Can you work these out from the model? Positions are in its coordinate system, mm. A direction names the side the tool comes from. Round coordinates to 2 decimals unless told otherwise and drop trailing zeros. Loops run counter-clockwise (first coordinate to the right, second up) from the corner with the lowest first, then second, coordinate; pieces in that order, holes last. Notation, with made-up numbers: (47.25, 21.25) -> (51.25, 21.25) arc R31 cw to (51.25, 50.25) -> close; hole circle Ø2 at (30.5, 84.5). An arc over 180 degrees is marked (long way). Answer as a JSON object with one key per item and string values.
```python
from build123d import *

# Parameters (mm, degrees)
F0_R     = 11.5502364961
F1_DEPTH = 76.2
F2_DEPTH = 25.4
F3_DEPTH = 25.4
F0_W     = 68.4429863468
F0_H     = 5.7512475178
F4_DEPTH = 76.2
F6_DEPTH = 25.4


with BuildPart() as f1:
    # F0 (on Top) → F1 (new body)
    with BuildSketch(Plane.XY):
        Polygon((-8.7633775547, 30.0670936704), (-48.5640950501, 30.0670936704), (-48.5640950501, -34.4098359346), (-8.7633775547, -34.4098359346), (-8.7633775547, -5.7512475178), (-8.7633775547, 0), align=None)
        with Locations((-30.1417633891, 0)):
            Circle(F0_R, mode=Mode.SUBTRACT)
    extrude(amount=F1_DEPTH)

    # F0 (on Top) → F2 (join)
    with BuildSketch(Plane.XY):
        Polygon((-8.7633775547, -5.7512475178), (-8.7633775547, -34.4098359346), (41.3302518427, -34.4098359346), (59.6796087921, -23.2587810606), (59.6796087921, -5.7512475178), align=None)
    extrude(amount=F2_DEPTH)

    # F0 (on Top) → F3 (join)
    with BuildSketch(Plane.XY):
        Polygon((41.3302518427, 30.0670936704), (-8.7633775547, 30.0670936704), (-8.7633775547, 0), (59.6796087921, 0), (59.6796087921, 18.9160387963), align=None)
    extrude(amount=F3_DEPTH)

    # F0 (on Top) → F4 (join)
    with BuildSketch(Plane.XY):
        with Locations((25.4581156187, -2.8756237589)):
            Rectangle(F0_W, F0_H)
    extrude(amount=F4_DEPTH)

    # F5 (on face) → F6 (cut)
    with BuildSketch(Plane.XZ.offset(5.7512475178)):
        Polygon((59.6796087921, 76.2), (-8.7633775547, 76.2), (59.6796087921, 25.4), align=None)
    extrude(amount=-F6_DEPTH, mode=Mode.SUBTRACT)


solid = f1.part
```
Q1. We'd pull the mould along X, two halves only. Please class faces 4 (the cylindrical face through (-39.308, -7.028, 37.567)), 5 (the flat face through (25, 15, 25.4)), 6 (the flat face through (-48.564, -2, 38)), 7 (the flat face through (-8.763, 15, 50)): pulls with the +X half, pulls with the -X half, needs draft (parallel to the pull), parting line crosses it, or undercut.
Determined:
{"face 4": "undercut", "face 5": "needs draft", "face 6": "pulls with the -X half", "face 7": "pulls with the +X half"}
Q2. I'm going to push flat-ended pins straight in: pin 1 (24 mm diameter, centred on y = 21.5, z = 42, fed in from +X); pin 2 (3 mm diameter, centred on x = 7, z = 62.5, fed in from -Y). Where does each tip first touch, or does it pass through?
Determined:
{"pin 1": "x = -8.76", "pin 2": "y = -5.75"}
Q3. I want a section at C-C, the plane y = -14.5. Write out the boundary of the cut face in (x, z), then the cut area to 3 significant figures.
Determined:
{"outline": "(-48.56, 0) -> (59.68, 0) -> (59.68, 25.4) -> (-8.76, 25.4) -> (-8.76, 76.2) -> (-48.56, 76.2) -> close", "area": "4,770 mm²"}
Q4. I want a section at D-D, the plane x = 27. Write out the boundary of the cut face in (y, z), then the cut area to 3 significant figures.
Determined:
{"outline": "(-34.41, 0) -> (30.07, 0) -> (30.07, 25.4) -> (0, 25.4) -> (0, 49.66) -> (-5.75, 49.66) -> (-5.75, 25.4) -> (-34.41, 25.4) -> close", "area": "1,780 mm²"}
Q5. I want a section at A-A, the plane y = -7.5. Write out the boundary of the cut face in (x, z), then the cut area to 3 significant figures.
Determined:
{"outline": "(-48.56, 0) -> (-38.93, 0) -> (-38.93, 76.2) -> (-48.56, 76.2) -> close; (-21.36, 0) -> (59.68, 0) -> (59.68, 25.4) -> (-8.76, 25.4) -> (-8.76, 76.2) -> (-21.36, 76.2) -> close", "area": "3,430 mm²"}
Q6. If I drill on L1, parallel to X at y = -15.5, z = 62.5; L2, parallel to Z at x = 21.5, y = 14.5; L3, parallel to X at y = -10, z = 25.5, over which ranges is the centre line in solid material (lowest first)? Write a range as [from, to].
Determined:
{"L1": "[-48.56, -8.76]", "L2": "[0, 25.4]", "L3": "[-48.56, -35.92], [-24.36, -8.76]"}
Q7. I want a section at B-B, the plane z = 39. Write out the boundary of the cut face in (x, y).
Determined:
{"outline": "(-48.56, -34.41) -> (-8.76, -34.41) -> (-8.76, -5.75) -> (41.36, -5.75) -> (41.36, 0) -> (-8.76, 0) -> (-8.76, 30.07) -> (-48.56, 30.07) -> close; hole circle Ø23.1 at (-30.14, 0)"}
Q8. On a 3-axis mill with a long thin cutter (end or side, diameter ignored), from which of +Z, -Z, +X, -X, +Y, -Y can I reach the whole of each face in a straight line? I mean faces 1 (the flat face through (17, 0, 45)), 2 (the flat face through (59.68, -2, 13)), 3 (the flat face through (25, -20, 25.4)). Say none if no direction works.
Determined:
{"face 1": "+Z, +X, +Y", "face 2": "+Z, -Z, +X, +Y, -Y", "face 3": "+Z, +X, -Y"}
